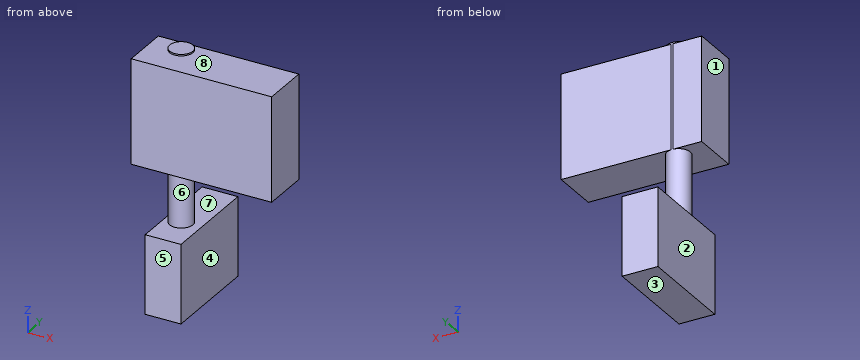
```python
from build123d import *

# Parameters (mm, degrees)
F0_W     = 190.5
F0_H     = 533.4
F1_DEPTH = 419.1
F2_R     = 61.948807
F3_DEPTH = 914.4
F4_W     = 747.836396
F4_H     = 555.345953
F5_DEPTH = 254


with BuildPart() as f1:
    # F0 (on Top) → F1 (new body)
    with BuildSketch(Plane.XY):
        with Locations((95.25, 266.7)):
            Rectangle(F0_W, F0_H)
    extrude(amount=F1_DEPTH)

    # F2 (on face) → F3 (join)
    with BuildSketch(Plane.XY.offset(419.1)):
        with Locations((82.928531, 192.244217)):
            Circle(F2_R)
    extrude(amount=F3_DEPTH)

    # F4 (on face) → F5 (join)
    with BuildSketch(Plane.XZ):
        with Locations((299.42248, 1047.925144)):
            Rectangle(F4_W, F4_H)
    extrude(amount=-F5_DEPTH)


solid = f1.part
```
Geometry check sheet. Reference: the model listing, model coordinates, mm. Face numbers are marked on the shaded views. A direction names the side the tool comes from. Coordinates: 2 decimals unless noted, no trailing zeros. Loops run counter-clockwise (first coordinate to the right, second up) from the corner with the lowest first, then second, coordinate; pieces in that order, holes last. Notation, with made-up numbers: (11, 56) -> (55, 56) arc R12 cw to (55, 77) -> close; hole circle Ø10 at (60.5, 23). An arc over 180 degrees is marked (long way). Put each result on its own line as item: value.
1) Cross-section at B-B on z = 950.5. Record the boundary of the cut face in (x, y).
Result set:
outline: (-74.5, 0) -> (673.34, 0) -> (673.34, 254) -> (87.82, 254) arc R61.95 ccw to (78.04, 254) -> (-74.5, 254) -> close
2) Tool access check on the marked faces 1, 2, 3 and 4. Record the directions out of +Z, -Z, +X, -X, +Y, -Y that give a thin tool (end or side, any length) a straight path to the whole face; none if there is none.
Result set:
face 1: +Z, -Z, -X, +Y, -Y
face 2: -Z, -X, +Y, -Y
face 3: -Z, +X, -X, +Y, -Y
face 4: -Z, +X, +Y, -Y
3) Cross-section at A-A on y = 83. Record the boundary of the cut face in (x, z), plus the area to 3 significant figures.
Result set:
outline: (-74.5, 770.25) -> (673.34, 770.25) -> (673.34, 1325.6) -> (-74.5, 1325.6) -> close; (0, 0) -> (190.5, 0) -> (190.5, 419.1) -> (0, 419.1) -> close
area: 495,000 mm^2
4) Cross-section at D-D on x = 370. Record the boundary of the cut face in (y, z).
Result set:
outline: (0, 770.25) -> (254, 770.25) -> (254, 1325.6) -> (0, 1325.6) -> close
5) Cross-section at C-C on y = 145.5. Record the boundary of the cut face in (x, z).
Result set:
outline: (-74.5, 770.25) -> (42.28, 770.25) -> (42.28, 419.1) -> (0, 419.1) -> (0, 0) -> (190.5, 0) -> (190.5, 419.1) -> (123.58, 419.1) -> (123.58, 770.25) -> (673.34, 770.25) -> (673.34, 1325.6) -> (123.58, 1325.6) -> (123.58, 1333.5) -> (42.28, 1333.5) -> (42.28, 1325.6) -> (-74.5, 1325.6) -> close
6) Gauge pin test, flat ends, axial feed: pin 1 Ø1 at (y, z) = (237, 442.5) entering from +X; pin 2 Ø1 at (x, z) = (31, 965.5) entering from +Y; pin 3 Ø8 at (x, y) = (68.5, 95.5) entering from -Z; pin 4 Ø10 at (y, z) = (292.5, 218) entering from +X. Record the tip position at first contact, or that the pin passes through.
Result set:
pin 1: stops at x = 126.28
pin 2: stops at y = 254
pin 3: stops at z = 0
pin 4: stops at x = 190.5
7) Release check for a two-part mould opening along Z. For the marked faces 5, 6, 7 and 8 record: released by +Z, released by -Z, zero draft, split by the parting line, or undercut.
Result set:
face 5: zero draft
face 6: undercut
face 7: undercut
face 8: released by +Z
8) Thickness scan on line 1 (Z direction, x = 484, y = 175); line 2 (X direction, y = 343.5, z = 257); line 3 (X direction, y = 192.5, z = 727). Record the ranges inside material, lowest first.
Result set:
line 1: z = 770.25 to 1325.6
line 2: x = 0 to 190.5
line 3: x = 20.98 to 144.88
